Drawing for the job (mm, zero at the part's lowest x, y, z). Give positions to 0.01 mm unless a question says otherwise; leave off trailing zeros. Order: outer loops, then holes, each group sorted by start corner. A loop starts at its lowest first (then second) coordinate and runs counter-clockwise, first axis right, second up. Notation, with made-up numbers: (62, 42) - (95, 42) arc R17 ccw to (95, 66) - close; hole circle Ø7 at (-1.75, -28). An arc over 180 degrees is marked (long way). Use a Markdown table: item, result.
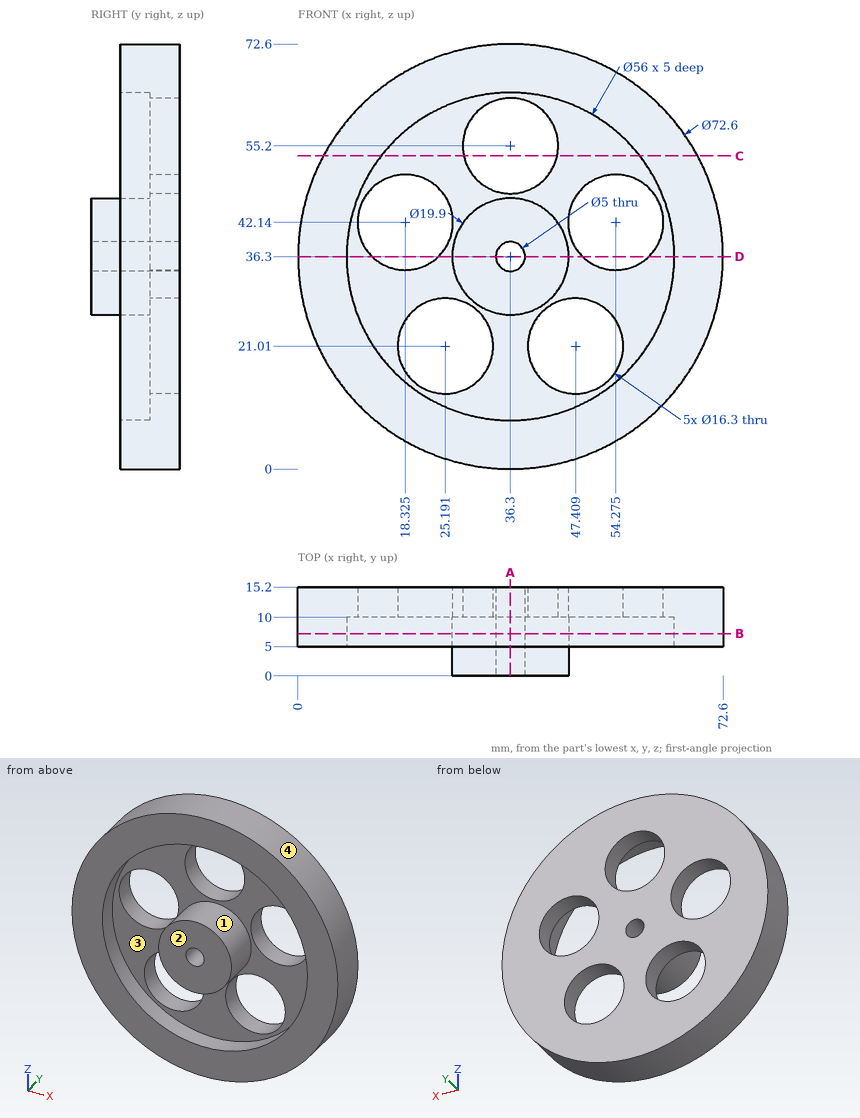
1) Slice it at C-C (z = 53.5). Write the cut outline in (x, y) (1 decimal), and give its area (3 significant figures).
Computed:
| item | result |
|---|---|
| outline | (4.3, 5) - (14.2, 5) - (14.2, 10) - (28.3, 10) - (28.3, 15.2) - (4.3, 15.2) - close; (44.3, 10) - (58.4, 10) - (58.4, 5) - (68.3, 5) - (68.3, 15.2) - (44.3, 15.2) - close |
| area | 348 mm² |
2) Pin check, flat tips, straight feed: P1, Ø1, axis at x = 48, z = 60.5, coming from the -Y side; P2, Ø3, axis at y = 9.5, z = 43.5, coming from the -X side; P3, Ø8, axis at x = 50.5, z = 60, coming from the -Y side. Stop position of each tip, or through.
Computed:
| item | result |
|---|---|
| P1 | stops at y = 10 |
| P2 | stops at x = 0.45 |
| P3 | stops at y = 5 |
3) Slice it at A-A (x = 36.3). Write the cut outline in (y, z).
Computed:
| item | result |
|---|---|
| outline | (0, 26.35) - (10, 26.35) - (10, 8.3) - (5, 8.3) - (5, 0) - (15.2, 0) - (15.2, 33.8) - (0, 33.8) - close; (0, 38.8) - (15.2, 38.8) - (15.2, 47.05) - (10, 47.05) - (10, 46.25) - (0, 46.25) - close; (5, 64.3) - (10, 64.3) - (10, 63.35) - (15.2, 63.35) - (15.2, 72.6) - (5, 72.6) - close |
4) Wall check: line 1 (Z direction, x = 36.3, y = 8.9); line 2 (Z direction, x = 22.5, y = 10.25) (1 decimal); line 3 (Z direction, x = 40.5, y = 5.25) (1 decimal). Give the ranges that are in metal, low to high. Write a range as from..to.
Computed:
| item | result |
|---|---|
| line 1 | z = 0..8.3, 26.35..33.8, 38.8..46.25, 64.3..72.6 |
| line 2 | z = 2.7..13.3, 28.7..35.1, 49.1..69.9 |
| line 3 | z = 0.2..8.6, 27.3..45.3, 64..72.4 |
5) Slice it at B-B (y = 7.25). Write the cut outline in (x, z).
Computed:
| item | result |
|---|---|
| outline | circle Ø72.6 at (36.3, 36.3); circle Ø19.9 at (36.3, 36.3); hole circle Ø56 at (36.3, 36.3); hole circle Ø5 at (36.3, 36.3) |
6) Two-plate mould, pull along Z, no slides. Class the marked faces 1, 2, 3 and 4: +Z half, -Z half, draft (parallel to the pull), parting line (faces both ways), or undercut.
Computed:
| item | result |
|---|---|
| face 1 | undercut |
| face 2 | draft |
| face 3 | undercut |
| face 4 | parting line |
7) Slice it at D-D (z = 36.3). Write the cut outline in (x, y), and give its area (3 significant figures).
Computed:
| item | result |
|---|---|
| outline | (0, 5) - (8.3, 5) - (8.3, 10) - (12.64, 10) - (12.64, 15.2) - (0, 15.2) - close; (24.01, 10) - (26.35, 10) - (26.35, 0) - (33.8, 0) - (33.8, 15.2) - (24.01, 15.2) - close; (38.8, 0) - (46.25, 0) - (46.25, 10) - (48.59, 10) - (48.59, 15.2) - (38.8, 15.2) - close; (59.96, 10) - (64.3, 10) - (64.3, 5) - (72.6, 5) - (72.6, 15.2) - (59.96, 15.2) - close |
| area | 465 mm² |
